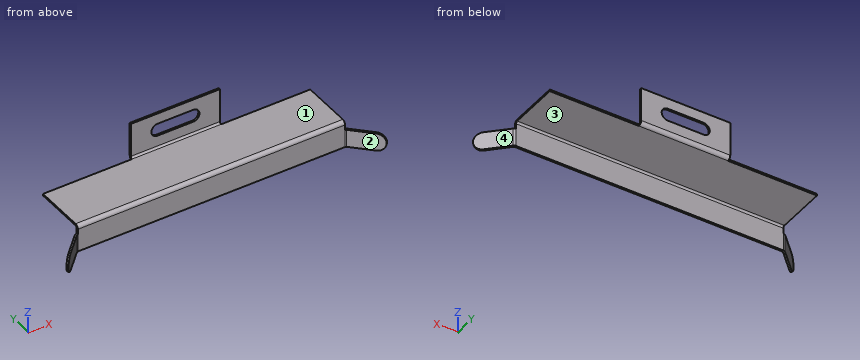
from build123d import *

# Parameters (mm, degrees)
CROQUIS1_W                       = 150
CROQUIS1_H                       = 30
BRIDA_BASE1_DEPTH                = 1
BRIDA_DE_ARISTA1_DEPTH           = 50
BRIDA_DE_ARISTA2_STRIP_W         = 6
BRIDA_DE_ARISTA2_STRIP_H         = 1
BRIDA_DE_ARISTA2_STRIP_CUT_DEPTH = 150
BRIDA_DE_ARISTA2_DEPTH           = 150
BRIDA_DE_ARISTA3_DEPTH           = 10
BRIDA_DE_ARISTA3_BEND_DEPTH      = 10
REDONDEO1_RADIUS                 = 5
REDONDEO1_LENGTH                 = 1
REDONDEO2_RADIUS                 = 5
REDONDEO2_LENGTH                 = 1
CORTAR_EXTRUIR1_DEPTH            = 10


# Sheet-metal steps are written as plain solids
with BuildPart() as part:
    # Croquis1 → Brida base1 (new body)
    with BuildSketch(Plane.XY):
        Rectangle(CROQUIS1_W, CROQUIS1_H)
    extrude(amount=-BRIDA_BASE1_DEPTH)

    # Brida de arista1 section (across the edge) → Brida de arista1 (add)
    with BuildSketch(Plane(origin=(25, 16, 0), x_dir=(0, -1, 0), z_dir=(-1, 0, 0))):
        with BuildLine():
            Line((-1, 1), (-1, 20))
            Line((-1, 20), (0, 20))
            Line((0, 20), (0, 1))
            ThreePointArc((0, 1), (0.292893219, 0.292893219), (1, 0))
            Line((1, 0), (1, -1))
            ThreePointArc((1, -1), (-0.414213562, -0.414213562), (-1, 1))
        make_face()
    extrude(amount=BRIDA_DE_ARISTA1_DEPTH)

    # Brida de arista2 strip (across the edge) → Brida de arista2 strip cut (cut)
    with BuildSketch(Plane(origin=(75, -15, -1), x_dir=(0, 1, 0), z_dir=(-1, 0, 0))):
        with Locations((-1, -0.5)):
            Rectangle(BRIDA_DE_ARISTA2_STRIP_W, BRIDA_DE_ARISTA2_STRIP_H)
    extrude(amount=BRIDA_DE_ARISTA2_STRIP_CUT_DEPTH, mode=Mode.SUBTRACT)

    # Brida de arista2 section (across the edge) → Brida de arista2 (add)
    with BuildSketch(Plane(origin=(75, -15, -1), x_dir=(0, 1, 0), z_dir=(-1, 0, 0))):
        with BuildLine():
            Line((0, 1), (0, 14))
            Line((0, 14), (1, 14))
            Line((1, 14), (1, 1))
            ThreePointArc((1, 1), (1.292893219, 0.292893219), (2, 0))
            Line((2, 0), (2, -1))
            ThreePointArc((2, -1), (0.585786438, -0.414213562), (0, 1))
        make_face()
    extrude(amount=BRIDA_DE_ARISTA2_DEPTH)

    # Brida de arista3 section (across the edge) → Brida de arista3 (add)
    with BuildSketch(Plane(origin=(-75.414213562, -15, -5), x_dir=(0.7071067811865439, -0.7071067811865511, 1.6984173230954452e-15), z_dir=(0, 0, -1))):
        with BuildLine():
            Line((-1, 0.414213562), (-1, 19.585786438))
            Line((-1, 19.585786438), (0, 19.585786438))
            Line((0, 19.585786438), (0, 0.414213562))
            ThreePointArc((0, 0.414213562), (0.076120467, 0.03153013), (0.292893219, -0.292893219))
            Line((0.292893219, -0.292893219), (-0.414213562, -1))
            ThreePointArc((-0.414213562, -1), (-0.847759065, -0.351153302), (-1, 0.414213562))
        make_face()
    extrude(amount=BRIDA_DE_ARISTA3_DEPTH)

    # Brida de arista3 section 2 (across the edge) → Brida de arista3 bend (add)
    with BuildSketch(Plane(origin=(75.414213562, -15, -15), x_dir=(-0.7071067811865437, -0.7071067811865513, 3.0194085743918815e-15), z_dir=(0, 0, 1))):
        with BuildLine():
            Line((-1, 0.414213562), (-1, 19.585786438))
            Line((-1, 19.585786438), (0, 19.585786438))
            Line((0, 19.585786438), (0, 0.414213562))
            ThreePointArc((0, 0.414213562), (0.076120467, 0.03153013), (0.292893219, -0.292893219))
            Line((0.292893219, -0.292893219), (-0.414213562, -1))
            ThreePointArc((-0.414213562, -1), (-0.847759065, -0.351153302), (-1, 0.414213562))
        make_face()
    extrude(amount=BRIDA_DE_ARISTA3_BEND_DEPTH)

    # Redondeo1: full round fillet: the end face becomes a half cylinder, R = half its width
    redondeo1_face = Plane((-89.617009358, -28.495689014, -10), x_dir=(-0.707106781187, 0.707106781187, 0), z_dir=(-0.707106781187, -0.707106781187, 0))  # on the end face: x along it, z out of the body
    redondeo1_slab = redondeo1_face.offset(-REDONDEO1_RADIUS / 2) * Box(REDONDEO1_LENGTH, 2 * REDONDEO1_RADIUS, REDONDEO1_RADIUS, mode=Mode.PRIVATE)  # the body's end, R deep
    redondeo1_round = Plane((-86.081475452, -24.960155108, -10), x_dir=(-0.707106781187, -0.707106781187, 0), z_dir=(-0.707106781187, 0.707106781187, 0)) * Cylinder(REDONDEO1_RADIUS, REDONDEO1_LENGTH, mode=Mode.PRIVATE)  # its axis R under the face
    add(redondeo1_slab - redondeo1_round, mode=Mode.SUBTRACT)

    # Redondeo2: full round fillet: the end face becomes a half cylinder, R = half its width
    redondeo2_face = Plane((89.617009358, -28.495689014, -10), x_dir=(0.707106781187, 0.707106781187, 0), z_dir=(0.707106781187, -0.707106781187, 0))  # on the end face: x along it, z out of the body
    redondeo2_slab = redondeo2_face.offset(-REDONDEO2_RADIUS / 2) * Box(REDONDEO2_LENGTH, 2 * REDONDEO2_RADIUS, REDONDEO2_RADIUS, mode=Mode.PRIVATE)  # the body's end, R deep
    redondeo2_round = Plane((86.081475452, -24.960155108, -10), x_dir=(0.707106781187, -0.707106781187, 0), z_dir=(0.707106781187, 0.707106781187, 0)) * Cylinder(REDONDEO2_RADIUS, REDONDEO2_LENGTH, mode=Mode.PRIVATE)  # its axis R under the face
    add(redondeo2_slab - redondeo2_round, mode=Mode.SUBTRACT)

    # Croquis18 → Cortar-Extruir1 (cut)
    with BuildSketch(Plane(origin=(0, 17, 0), x_dir=(1, 0, 0), z_dir=(0, 1, 0))):
        with BuildLine():
            Line((10, -14), (-10, -14))
            ThreePointArc((-10, -14), (-13.5, -10.5), (-10, -7))
            Line((-10, -7), (10, -7))
            ThreePointArc((10, -7), (13.5, -10.5), (10, -14))
        make_face()
    extrude(amount=-CORTAR_EXTRUIR1_DEPTH, mode=Mode.SUBTRACT)


solid = part.part
Design review of the part built by this model. Coordinates are the model's own, in mm. Face numbers are marked on the shaded views. A direction names the side the tool comes from. Coordinates: 2 decimals unless noted, no trailing zeros. Loops run counter-clockwise (first coordinate to the right, second up) from the corner with the lowest first, then second, coordinate; pieces in that order, holes last. Notation, with made-up numbers: (41.5, 79.5) -> (70.5, 79.5) arc R19 ccw to (70.5, 99.5) -> close; hole circle Ø10 at (-24.75, 60.25). An arc over 180 degrees is marked (long way). Use a Markdown table: item, result. Add a question column.
Item 1: Clearance check with flat-ended pins moving along their axes: P1, Ø0.5, axis at x = -57, z = -0.5, coming from the +Y side; P2, Ø12, axis at x = 6, z = 10, coming from the -Y side; P3, Ø4, axis at x = -54, y = 1, coming from the -Z side; P4, Ø4, axis at y = 7.5, z = -3.5, coming from the -X side. State where each tip first meets the part, or that it passes through.
Item 2: We need section C-C, the plane x = 73. Write out the cut boundary in (y, z).
Item 3: We need section D-D, the plane z = -8. Write out the cut boundary in (x, y), and give its area (3 significant figures).
Item 4: We need section A-A, the plane z = 10.5. Write out the cut boundary in (x, y), and give its area (3 significant figures).
Item 5: Wall thickness on L1, parallel to Z at x = -24, y = -3.5; L2, parallel to Y at x = 8, z = 15.5; L3, parallel to Y at x = 11, z = -12.5: over which ranges is each line inside the solid? List them lowest first. Write a range as from..to.
Item 6: We need section B-B, the plane y = -19.5. Write out the cut boundary in (x, z), and give its area (3 significant figures).
Item 7: Machinability: for the marked faces 1, 2, 3 and 4, which of the approach directions +Z, -Z, +X, -X, +Y, -Y give a long, thin tool a straight path to every point of the face, cutting with its end or side? Answer none if there is none.
Numbers:
| question | item | result |
|---|---|---|
| 1 | P1 | stops at y = 15 |
| 1 | P2 | stops at y = 16 |
| 1 | P3 | stops at z = -1 |
| 1 | P4 | passes through |
| 2 | outline | (-15, -15) -> (-14, -15) -> (-14, -2) arc R1 cw to (-13, -1) -> (15, -1) -> (15, 0) -> (-13, 0) arc R2 ccw to (-15, -2) -> close |
| 3 | outline | (-89.68, -27.85) -> (-88.97, -28.55) -> (-75.71, -15.29) arc R1 cw to (-75, -15) -> (75, -15) arc R1 cw to (75.71, -15.29) -> (88.97, -28.55) -> (89.68, -27.85) -> (76.41, -14.59) arc R2 ccw to (75, -14) -> (-75, -14) arc R2 ccw to (-76.41, -14.59) -> close |
| 3 | area | 190 mm^2 |
| 4 | outline | (-25, 16) -> (-13.5, 16) -> (-13.5, 17) -> (-25, 17) -> close; (13.5, 16) -> (25, 16) -> (25, 17) -> (13.5, 17) -> close |
| 4 | area | 23.0 mm^2 |
| 5 | L1 | z = -1..0 |
| 5 | L2 | y = 16..17 |
| 5 | L3 | y = -15..-14 |
| 6 | outline | (-81.33, -15) -> (-79.91, -15) -> (-79.91, -5) -> (-81.33, -5) -> close; (79.91, -15) -> (81.33, -15) -> (81.33, -5) -> (79.91, -5) -> close |
| 6 | area | 28.3 mm^2 |
| 7 | face 1 | +Z, +X, -X, -Y |
| 7 | face 2 | +Z, -Z, -Y |
| 7 | face 3 | -Z, +X, -X, +Y |
| 7 | face 4 | +Z, -Z, +X, +Y |
